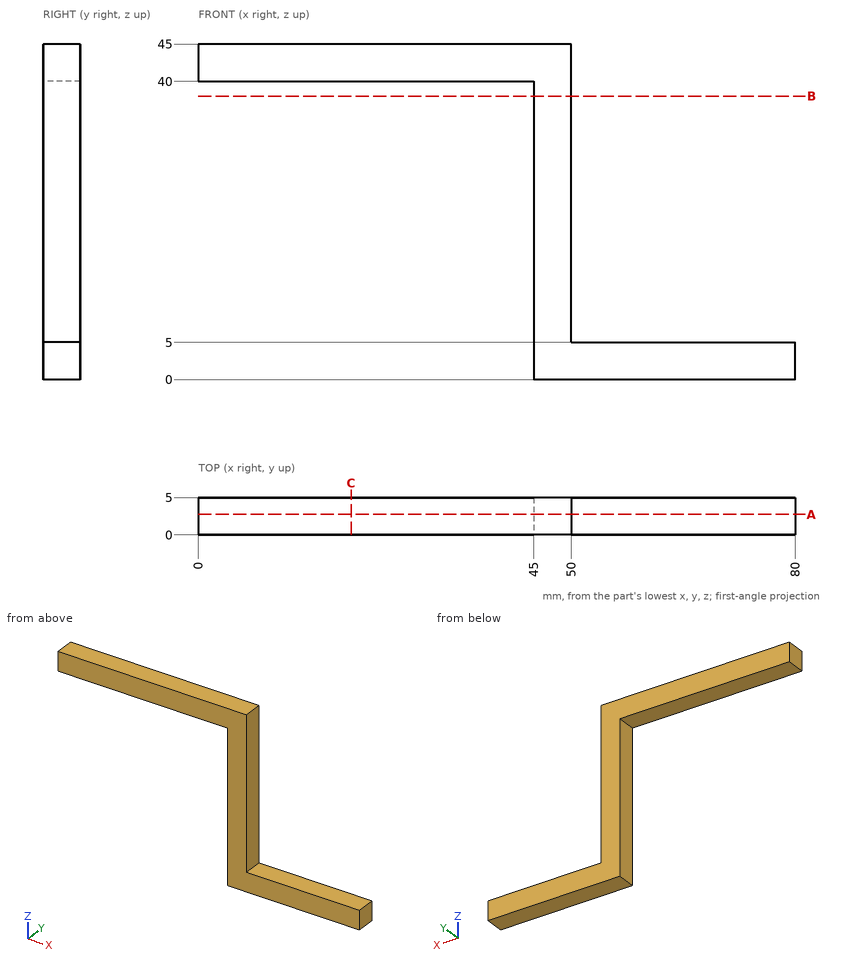
Geometry: see drawing. Coordinates: mm, zero at the bounding-box minimum. Coordinates: 2 decimals unless noted, no trailing zeros. Loops run counter-clockwise (first coordinate to the right, second up) from the corner with the lowest first, then second, coordinate; pieces in that order, holes last.
(1) Section A-A on y = 2.75. Return the cut outline in (x, z), then the cut area to 3 significant figures.
(2) Section C-C on x = 20.5. Return the cut outline in (y, z).
(3) Material intervals for probe 1 along X at (y, z) = (4.7, 15.5); probe 2 along Z at (x, y) = (27, 3.75); probe 3 along Z at (x, y) = (74, 3.15), sorted ascending.
(4) First-contact query: pin 1 Ø2.5 at (y, z) = (2.5, 22) entering from -X; pin 2 Ø2 at (x, y) = (38, 1.5) entering from -Z; pin 3 Ø2 at (y, z) = (1.5, 10.5) entering from +X. Flat tips, straight axial feed; report the tip coordinate or a pass-through.
(5) Section B-B on z = 38. Return the cut outline in (x, y).
Data:
1. outline: (0, 40) - (45, 40) - (45, 0) - (80, 0) - (80, 5) - (50, 5) - (50, 45) - (0, 45) - close
1. area: 600 mm2
2. outline: (0, 40) - (5, 40) - (5, 45) - (0, 45) - close
3. probe 1: x = 45 to 50
3. probe 2: z = 40 to 45
3. probe 3: z = 0 to 5
4. pin 1: stops at x = 45
4. pin 2: stops at z = 40
4. pin 3: stops at x = 50
5. outline: (45, 0) - (50, 0) - (50, 5) - (45, 5) - close
